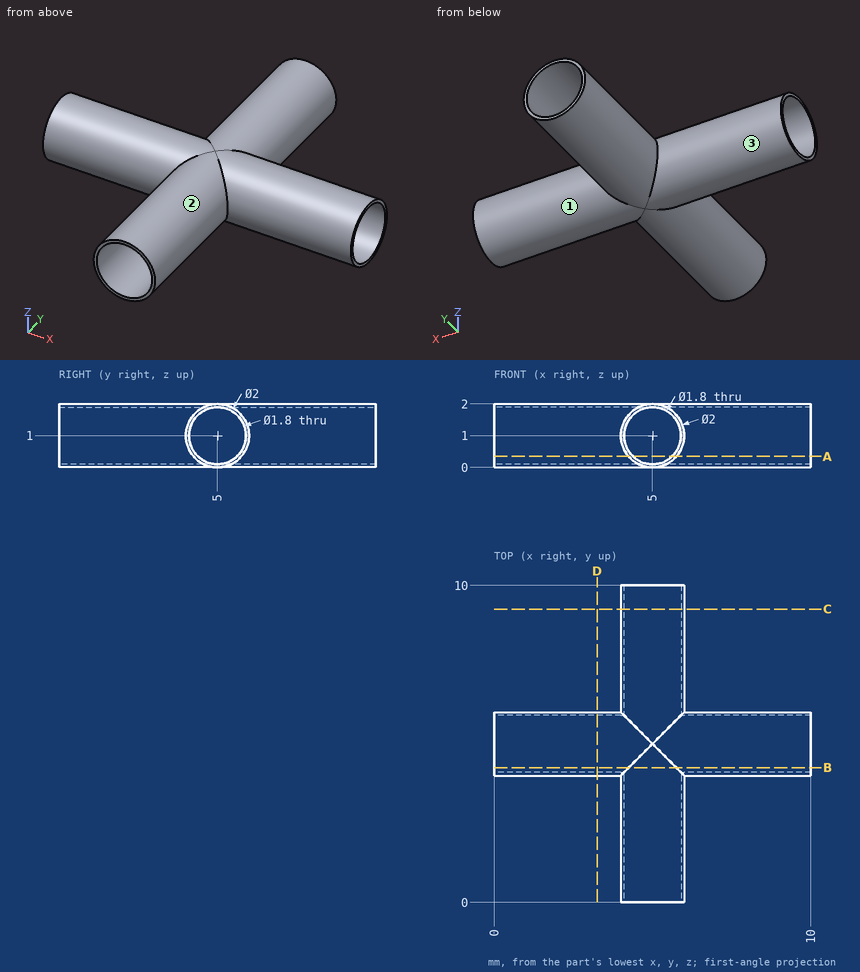
Design review of the part shown in the three views and the two pictorial views. Dimensions are in mm from the part's minimum x, y and z. A direction names the side the tool comes from. Round coordinates to 2 decimals unless told otherwise and drop trailing zeros. Order: outer loops, then holes, each group sorted by start corner. A loop starts at its lowest first (then second) coordinate and runs counter-clockwise, first axis right, second up. Notation, with made-up numbers: M 73.5,-12 L 108.5,-12 A12 ccw 108.5,-2 Z; hole C -1,-17.75 d4. An arc over 180 degrees is marked long. Put each result on its own line as item: value.
Q1. Consider section C-C (y = 9.25). State the section outline as (x, z) points.
Reported:
outline: C 5,1 d2; hole C 5,1 d1.8
Q2. Insertion check: pin 1 Ø4 at (x, y) = (8.5, 8.5) entering from -Z. The pin has a flat end and moves straight along its axis. Give the tip position at first contact, or say it passes through.
Reported:
pin 1: through
Q3. To check wall thickness, follow line 1 (Y direction, x = 3, z = 1.8); line 2 (Z direction, x = 4.25, y = 2). State the ranges of each line that lie inside material, in increasing order.
Reported:
line 1: 4.4 to 4.59, 5.41 to 5.6
line 2: 0.34 to 0.5, 1.5 to 1.66
Q4. Machinability: for the marked faces 1, 2 and 3, which of the approach directions +Z, -Z, +X, -X, +Y, -Y give a long, thin tool a straight path to every point of the face, cutting with its end or side? Answer none if there is none.
Reported:
face 1: +X
face 2: -Y
face 3: -X
Q5. Consider section A-A (z = 0.35). State the section outline as (x, y) points.
Reported:
outline: M 0,4.24 L 4.24,4.24 L 4.24,0 L 4.38,0 L 4.38,4.38 L 0,4.38 Z; M 0,5.62 L 4.38,5.62 L 4.38,10 L 4.24,10 L 4.24,5.76 L 0,5.76 Z; M 5.62,0 L 5.76,0 L 5.76,4.24 L 10,4.24 L 10,4.38 L 5.62,4.38 Z; M 5.62,5.62 L 10,5.62 L 10,5.76 L 5.76,5.76 L 5.76,10 L 5.62,10 Z
Q6. Consider section B-B (y = 4.25). State the section outline as (x, z) points, and give its area (3 significant figures).
Reported:
outline: M 0,0.34 L 4.25,0.34 A1 ccw 5.75,0.34 L 10,0.34 L 10,0.5 L 5.75,0.5 A0.9 cw 4.25,0.5 L 0,0.5 Z; M 0,1.5 L 4.25,1.5 A0.9 cw 5.75,1.5 L 10,1.5 L 10,1.66 L 5.75,1.66 A1 ccw 4.25,1.66 L 0,1.66 Z
area: 3.13 mm²
